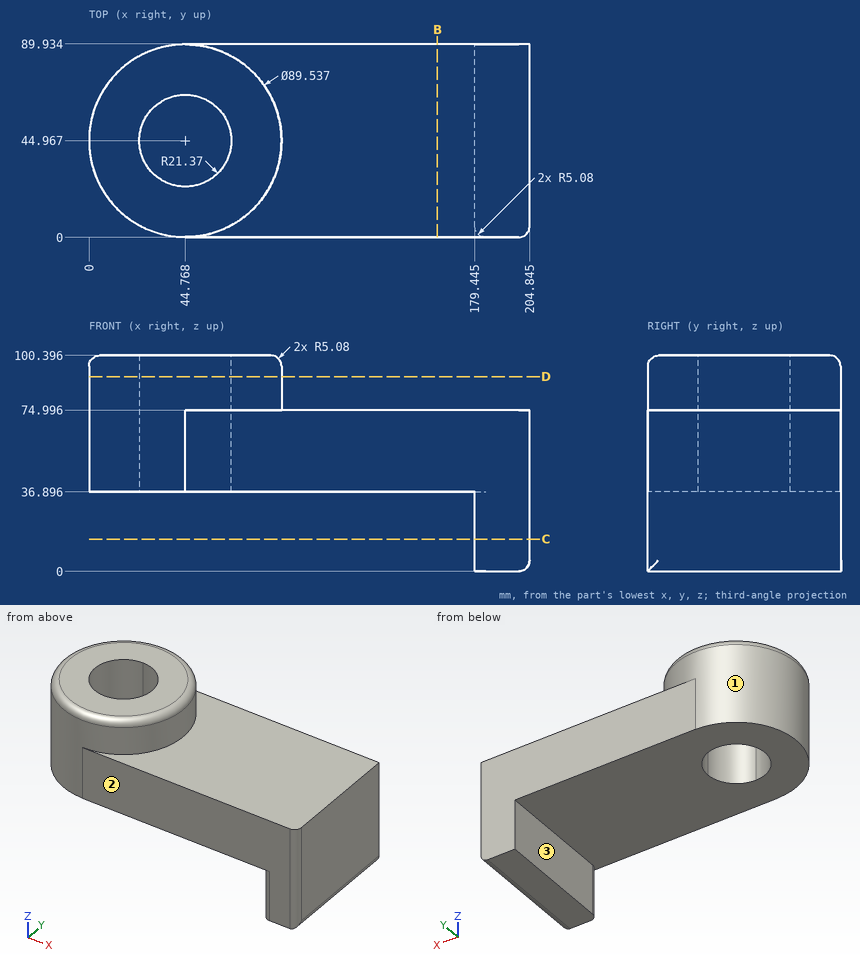
Geometry check sheet. Reference: drawing and pictorial views, mm from the part's lowest x, y, z. A direction names the side the tool comes from. Coordinates: 2 decimals unless noted, no trailing zeros. Order: outer loops, then holes, each group sorted by start corner. A loop starts at its lowest first (then second) coordinate and runs counter-clockwise, first axis right, second up. Notation, with made-up numbers: (62.25, 1.25) - (111.25, 1.25) arc R23 cw to (111.25, 20.25) - close; hole circle Ø10 at (0, -37.75). An arc over 180 degrees is marked (long way). Answer in a Markdown table with one row per item. Add a question column.
1) Gauge pin test, flat ends, axial feed: P1, Ø8, axis at x = 148, y = 9.5, coming from the +Z side; P2, Ø8, axis at y = 72, z = 78.5, coming from the +X side (1 decimal); P3, Ø6, axis at x = 36.5, z = 51.5, coming from the -Y side; P4, Ø6, axis at y = 60, z = 34, coming from the -X side. Record the tip position at first contact, or that the pin passes through.
2) Material ranges on line 1 along Z through (x, y) = (36, 14) (1 decimal); line 2 along Z through (x, y) = (151, 31.5) (1 decimal); line 3 along X through (y, z) = (31, 45) (1 decimal), recorded low to high. Write a range as [from, to].
3) Cross-section at C-C, the plane z = 15. Record the cut outline in (x, y) (1 decimal).
4) Cross-section at B-B, the plane x = 162. Record the cut outline in (y, z) (1 decimal).
5) Set-up check for the marked faces 1, 2 and 3: record each of +Z, -Z, +X, -X, +Y, -Y from which the full face is reachable in a straight line by a thin tool's end or side.
6) Cross-section at D-D, the plane z = 90.5. Record the cut outline in (x, y), then the cut area to 3 significant figures.
Check result:
| question | item | result |
|---|---|---|
| 1 | P1 | stops at z = 75 |
| 1 | P2 | stops at x = 204.8 |
| 1 | P3 | stops at y = 0.51 |
| 1 | P4 | stops at x = 2.33 |
| 2 | line 1 | z = [36.9, 100.4] |
| 2 | line 2 | z = [36.9, 75] |
| 2 | line 3 | x = [2.2, 28.6], [60.9, 204.8] |
| 3 | outline | (179.4, 5.1) arc R5.1 ccw to (184.5, 0) - (199.8, 0) arc R5.1 ccw to (204.8, 5.1) - (204.8, 89.9) - (179.4, 89.9) - close |
| 4 | outline | (0, 36.9) - (89.9, 36.9) - (89.9, 75) - (0, 75) - close |
| 5 | face 1 | +Z |
| 5 | face 2 | +Z, -Z, +X, -X, -Y |
| 5 | face 3 | -Z, -X, +Y, -Y |
| 6 | outline | circle Ø89.54 at (44.77, 44.97); hole circle Ø42.74 at (44.77, 44.97) |
| 6 | area | 4,860 mm² |
